Autodesk Inventor part; units mm, degrees
ref_plane "YZ Plane" through (0, 0, 0) normal (1, 0, 0) x (0, 1, 0)
ref_plane "XZ Plane" through (0, 0, 0) normal (0, 1, 0) x (-1, 0, 0)
ref_plane "XY Plane" through (0, 0, 0) normal (0, 0, 1) x (1, 0, 0)
sketch "Sketch1" plane through (0, 0, 0) normal (1, 0, 0) x (0, 1, 0)
  line L0 (5, 20) -> (-5, 20)
  line L1 (5, -20) -> (-5, -20)
  arc A0 (5, -24.4949) -> (5, 24.4949) centre (0, 0) ccw
  arc A1 (-5, 24.4949) -> (-5, -24.4949) centre (0, 0) ccw
  line L2 (5, 24.4949) -> (5, 20)
  line L3 (5, -20) -> (5, -24.4949)
  line L4 (-5, -24.4949) -> (-5, -20)
  line L5 (-5, 20) -> (-5, 24.4949)
  dimension "d3" = 20
  dimension "d4" = 40
  dimension "d7" = 25
  dimension "d8" = 25
  dimension "d9" = 10
extrude "Extrusion1" add sketch "Sketch1" along normal blind 156
properties part number "SpinnerAxelV1"
Geometry check sheet. Reference: the model listing, model coordinates, mm. A direction names the side the tool comes from. Coordinates: 2 decimals unless noted, no trailing zeros. Order: outer loops, then holes, each group sorted by start corner. A loop starts at its lowest first (then second) coordinate and runs counter-clockwise, first axis right, second up. Notation, with made-up numbers: M 44,22 L 56,22 A24 ccw 56,39 Z; hole C 60.25,81 d6. An arc over 180 degrees is marked long. Use CSV: the item, a comma, the result in double quotes.
Item 1: Mould release check, pull along Y, two halves, no side actions. Record for faces 4 (the flat face through (77, -5, -22)), 5 (the cylindrical face through (77, 25, 0)), 6 (the flat face through (156, 0, 0)): pulls with the +Y half, pulls with the -Y half, needs draft (parallel to the pull), parting line crosses it, or undercut.
Returned:
face 4,"undercut"
face 5,"pulls with the +Y half"
face 6,"needs draft"
Item 2: Thickness scan on line 1 along Z through (x, y) = (71, 3.5); line 2 along Y through (x, z) = (148.5, -5). Record the ranges inside material, lowest first.
Returned:
line 1,"z = -20 to 20"
line 2,"y = -24.49 to 24.49"
Item 3: Cross-section at C-C on y = 3.5. Record the cut outline in (x, z).
Returned:
outline,"M 0,-20 L 156,-20 L 156,20 L 0,20 Z"
Item 4: Cross-section at A-A on x = 144. Record the cut outline in (y, z).
Returned:
outline,"M -5,-24.49 L -5,-20 L 5,-20 L 5,-24.49 A25 ccw 5,24.49 L 5,20 L -5,20 L -5,24.49 A25 ccw Z"
Item 5: Gauge pin test, flat ends, axial feed: pin 1 Ø1.5 at (y, z) = (15, -17.5) entering from -X; pin 2 Ø2 at (x, z) = (85.5, -21.5) entering from -Y; pin 3 Ø2 at (x, z) = (84, 21.5) entering from +Y; pin 4 Ø3.5 at (x, z) = (81, -22) entering from +Y. Record the tip position at first contact, or that the pin passes through.
Returned:
pin 1,"stops at x = 0"
pin 2,"stops at y = -14.31"
pin 3,"stops at y = 14.31"
pin 4,"stops at y = 14.66"
Item 6: Tool access check on faces 1 (the flat face through (77, 0, -20)), 2 (the cylindrical face through (77, -25, 0)), 3 (the flat face through (77, -5, 22)). Record the directions out of +Z, -Z, +X, -X, +Y, -Y that give a thin tool (end or side, any length) a straight path to the whole face; none if there is none.
Returned:
face 1,"-Z, +X, -X"
face 2,"+X, -X, -Y"
face 3,"+Z, +X, -X"
Item 7: Cross-section at B-B on z = 5. Record the cut outline in (x, y), then the cut area to 3 significant figures.
Returned:
outline,"M 0,-24.49 L 156,-24.49 L 156,24.49 L 0,24.49 Z"
area,"7,640 mm2"
